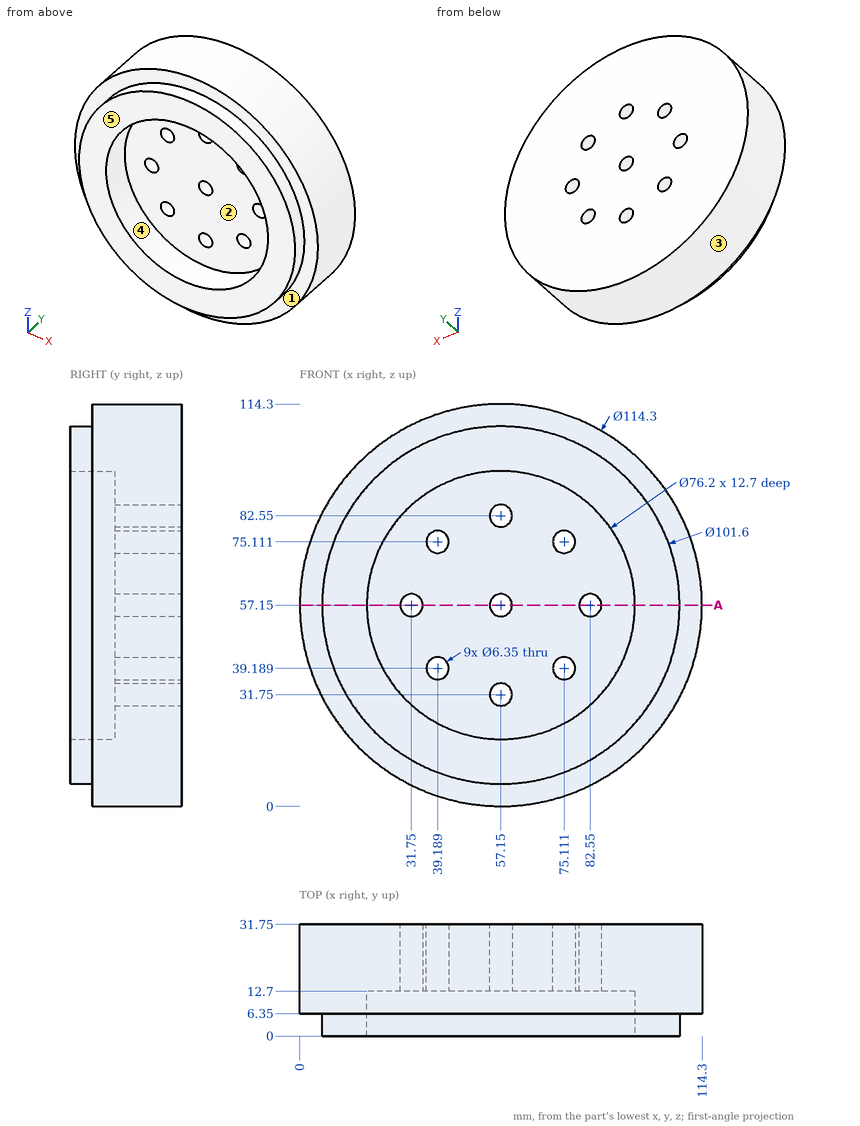
Design review of the part shown in the three views and the two pictorial views. Dimensions are in mm from the part's minimum x, y and z. A direction names the side the tool comes from. Give positions to 0.01 mm unless a question says otherwise; leave off trailing zeros.
(1) Wall thickness on line 1 along X through (y, z) = (22, 57); line 2 along Z through (x, y) = (57.15, 21) (1 decimal); line 3 along X through (y, z) = (30, 56): over which ranges is each line inside the solid? List them lowest first.
Checked values:
line 1: x = 0 to 28.58, 34.92 to 53.98, 60.32 to 79.38, 85.72 to 114.3
line 2: z = 0 to 28.6, 34.9 to 54, 60.3 to 79.4, 85.7 to 114.3
line 3: x = 0.01 to 28.79, 34.71 to 54.19, 60.11 to 79.59, 85.51 to 114.29
(2) Clearance check with flat-ended pins moving along their axes: pin 1 Ø12 at (y, z) = (20, 71.5) entering from +X; pin 2 Ø8.5 at (x, z) = (57.15, 57.15) entering from -Y; pin 3 Ø7.5 at (x, z) = (75.11, 75.11) entering from +Y; pin 4 Ø4 at (x, z) = (75.11, 39.19) entering from +Y. State where each tip first meets the part, or that it passes through.
Checked values:
pin 1: stops at x = 113.69
pin 2: stops at y = 12.7
pin 3: stops at y = 31.75
pin 4: passes through
(3) Mouldability with a two-part tool opening along X and no side actions: class the marked faces 1, 2 and 3 as +X half, -X half, draft (parallel to the pull), parting line (faces both ways), or undercut.
Checked values:
face 1: draft
face 2: undercut
face 3: parting line
(4) Add section A-A (z = 57.15). Give the number of separate pieces and of enclosed holes in the cut face, and give its area (3 significant figures).
Checked values:
separate pieces: 4
enclosed holes: 0
area: 2,220 mm2
(5) Tool access review of the marked faces 4 and 5: name each direction out of +Z, -Z, +X, -X, +Y, -Y from which nothing blocks a thin tool from reaching the whole face with its end or side.
Checked values:
face 4: -Y
face 5: +Z, -Z, +X, -X, -Y
